```python
from build123d import *

# Parameters (mm, degrees)
BOSS_EXTRUDE1_DEPTH = 12.5
SKETCH2_R           = 6.25
SKETCH2_R_2         = 2.4
BOSS_EXTRUDE2_DEPTH = 4.4
SKETCH3_R           = 2.4
BOSS_EXTRUDE3_DEPTH = 3.2
SKETCH4_R           = 1.25
CUT_EXTRUDE1_DEPTH  = 3.2
CUT_EXTRUDE2_DEPTH  = 3.2


with BuildPart() as part:
    # Sketch1 → Boss-Extrude1 (new body)
    with BuildSketch(Plane(origin=(0, 0, 0), x_dir=(1, 0, 0), z_dir=(0, 1, 0))):
        Polygon((-7.197362046, -11.706627962), (15.14596589, -17.163339125), (18.941938873, -1.620154473), (24.284908597, -2.925020186), (24.854304545, -0.593542489), (19.511334821, 0.711323224), (20.555227391, 4.985699003), (-1.788100545, 10.442410167), (-2.831993116, 6.168034388), (-8.17496284, 7.472900101), (-8.744358787, 5.141422403), (-3.401389063, 3.83655669), align=None)
    extrude(amount=BOSS_EXTRUDE1_DEPTH)

    # Sketch2 → Boss-Extrude2 (add)
    with BuildSketch(Plane(origin=(2.306064383, 0, -9.442528881), x_dir=(-0.971449041, 0, -0.237248311), z_dir=(0.237248311, 0, -0.971449041))):
        with Locations((-2.035507261, 6.25)):
            Circle(SKETCH2_R)
        with Locations((-8.285507261, 6.25)):
            Circle(SKETCH2_R_2)
    extrude(amount=BOSS_EXTRUDE2_DEPTH)

    # Sketch3 → Boss-Extrude3 (add)
    with BuildSketch(Plane(origin=(3.349956953, 0, -13.71690466), x_dir=(-0.971449041, 0, -0.237248311), z_dir=(0.237248311, 0, -0.971449041))):
        with Locations((-2.035507261, 6.25)):
            Circle(SKETCH3_R)
    extrude(amount=BOSS_EXTRUDE3_DEPTH)

    # Sketch4 → Cut-Extrude1 (cut)
    with BuildSketch(Plane(origin=(1.262171813, 0, -5.168153102), x_dir=(-0.971449041, 0, -0.237248311), z_dir=(0.237248311, 0, -0.971449041))):
        with Locations((-21.435507261, 6.25)):
            Circle(SKETCH4_R)
        Polygon((-24.285507261, 6.25), (-24.285507261, 6.75), (-22.581151185, 6.75), (-22.581151185, 5.75), (-24.285507261, 5.75), align=None)
    extrude(amount=-CUT_EXTRUDE1_DEPTH, mode=Mode.SUBTRACT)

    # Sketch5 → Cut-Extrude2 (cut)
    with BuildSketch(Plane(origin=(1.262171813, 0, -5.168153102), x_dir=(-0.971449041, 0, -0.237248311), z_dir=(0.237248311, 0, -0.971449041))):
        with BuildLine():
            ThreePointArc((8.358804544, 6.75), (6.611198873, 7.805252387), (5.288749178, 6.25))
            Line((5.288749178, 6.25), (6.864492739, 6.25))
            Line((6.864492739, 6.25), (7.879253637, 6.25))
            Line((7.879253637, 6.25), (7.879253637, 6.75))
            Line((7.879253637, 6.75), (8.358804544, 6.75))
        make_face()
        with BuildLine():
            Line((6.864492739, 6.25), (5.288749178, 6.25))
            ThreePointArc((5.288749178, 6.25), (6.611198873, 4.694747613), (8.358804544, 5.75))
            Line((8.358804544, 5.75), (7.879253637, 5.75))
            Line((7.879253637, 5.75), (7.879253637, 6.25))
            Line((7.879253637, 6.25), (6.864492739, 6.25))
        make_face()
        with BuildLine():
            ThreePointArc((8.4402363, 6.25), (8.419745126, 5.996706134), (8.358804544, 5.75))
            Line((8.358804544, 5.75), (9.714492739, 5.75))
            Line((9.714492739, 5.75), (9.714492739, 6.25))
            Line((9.714492739, 6.25), (8.4402363, 6.25))
        make_face()
        with BuildLine():
            Line((9.714492739, 6.75), (8.358804544, 6.75))
            ThreePointArc((8.358804544, 6.75), (8.419745126, 6.503293866), (8.4402363, 6.25))
            Line((8.4402363, 6.25), (9.714492739, 6.25))
            Line((9.714492739, 6.25), (9.714492739, 6.75))
        make_face()
        with BuildLine():
            ThreePointArc((8.4402363, 6.25), (8.419745126, 6.503293866), (8.358804544, 6.75))
            Line((8.358804544, 6.75), (7.879253637, 6.75))
            Line((7.879253637, 6.75), (7.879253637, 6.25))
            Line((7.879253637, 6.25), (8.4402363, 6.25))
        make_face()
        with BuildLine():
            Line((7.879253637, 5.75), (8.358804544, 5.75))
            ThreePointArc((8.358804544, 5.75), (8.419745126, 5.996706134), (8.4402363, 6.25))
            Line((8.4402363, 6.25), (7.879253637, 6.25))
            Line((7.879253637, 6.25), (7.879253637, 5.75))
        make_face()
    extrude(amount=-CUT_EXTRUDE2_DEPTH, mode=Mode.SUBTRACT)


solid = part.part
```
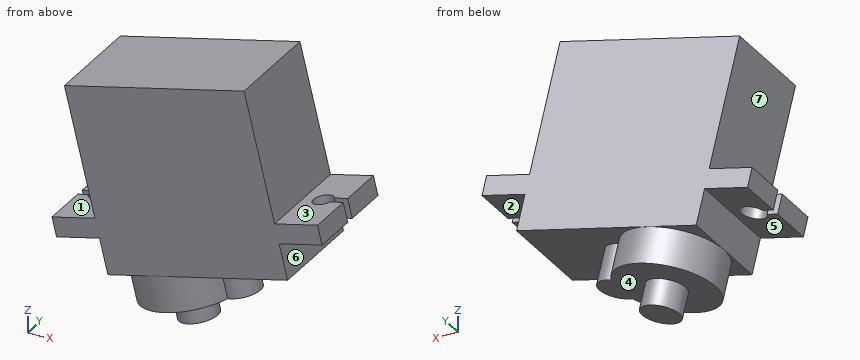
Design review of the part built by this model. Coordinates are the model's own, in mm. Face numbers are marked on the shaded views. A direction names the side the tool comes from. Coordinates: 2 decimals unless noted, no trailing zeros. Loops run counter-clockwise (first coordinate to the right, second up) from the corner with the lowest first, then second, coordinate; pieces in that order, holes last. Notation, with made-up numbers: M 44.25,-13 L 88.25,-13 A13 cw 88.25,5 Z; hole C 15.25,-26.75 d3. An arc over 180 degrees is marked long. One line per question, with ' | ' between items.
(1) We need section C-C (z = 10.5). Give the boundary of the cut face in (x, y).
Filled in:
outline: M -6.9,0 L 16.77,0 L 16.77,12.5 L -6.9,12.5 Z
(2) We need section A-A (y = 10.75). Give the boundary of the cut face in (x, z), and give its area (3 significant figures).
Filled in:
outline: M -8.74,-5.14 L -8.17,-7.47 L -2.83,-6.17 L -1.79,-10.44 L 0.07,-9.99 L 1.11,-14.26 L 9.54,-12.2 L 8.5,-7.93 L 20.56,-4.99 L 19.51,-0.71 L 24.85,0.59 L 24.28,2.93 L 18.94,1.62 L 15.15,17.16 L -7.2,11.71 L -3.4,-3.84 Z | area: 589 mm^2
(3) We need section B-B (z = 14). Give the boundary of the cut face in (x, y).
Filled in:
outline: M 2.19,0 L 15.92,0 L 15.92,12.5 L 2.19,12.5 Z
(4) Draft analysis for pull direction X (two halves, no side actions). For the marked faces 1, 2, 3 and 4, state which applies: released by +X, released by -X, zero draft, split by the parting line, or undercut.
Filled in:
face 1: released by -X | face 2: released by +X | face 3: undercut | face 4: undercut
(5) For pin 1 Ø1 at (x, y) = (7, 1.5) entering from -Z; pin 2 Ø2 at (y, z) = (10, 4.5) entering from +X; pin 3 Ø4 at (y, z) = (7, 5.5) entering from -X, all flat-tipped, find the tip position at first contact; note any pin that passes through.
Filled in:
pin 1: stops at z = -12.95 | pin 2: stops at x = 18.48 | pin 3: stops at x = -6.17
(6) Wall thickness on probe 1 along X at (y, z) = (10.5, 3); probe 2 along Z at (x, y) = (1, 6.5); probe 3 along X at (y, z) = (2.5, -9): over which ranges is each line inside the solid? List them lowest first.
Filled in:
probe 1: x = -5.07 to 18.6 | probe 2: z = -14.29 to 13.71 | probe 3: x = -2.14 to 9.44
(7) Machinability: for the marked faces 5, 6 and 7, which of the approach directions +Z, -Z, +X, -X, +Y, -Y give a long, thin tool a straight path to every point of the face, cutting with its end or side? Answer none if there is none.
Filled in:
face 5: -Z, +Y, -Y | face 6: +X, +Y, -Y | face 7: -X, +Y, -Y
